```python
from build123d import *

# Parameters (mm, degrees)
SKETCH1_R           = 4.25
BOSS_EXTRUDE1_DEPTH = 20
SKETCH2_R           = 1
BOSS_EXTRUDE2_DEPTH = 0.5
SKETCH3_R           = 0.5
BOSS_EXTRUDE3_DEPTH = 5
FILLET2_R           = 0.5
FILLET3_R           = 0.1
FILLET4_R           = 0.5


with BuildPart() as part:
    # Sketch1 → Boss-Extrude1 (new body)
    with BuildSketch(Plane.XY):
        Circle(SKETCH1_R)
    extrude(amount=BOSS_EXTRUDE1_DEPTH)

    # Sketch2 → Boss-Extrude2 (add)
    with BuildSketch(Plane.XY.offset(20)):
        Circle(SKETCH2_R)
    extrude(amount=BOSS_EXTRUDE2_DEPTH)

    # Sketch3 → Boss-Extrude3 (add)
    with BuildSketch(Plane.XY.offset(20.5)):
        Circle(SKETCH3_R)
    extrude(amount=BOSS_EXTRUDE3_DEPTH)

    # Fillet2
    fillet2_edges = [part.edges().sort_by_distance(p)[0] for p in [
        (-4.25, 0, 20),
    ]]
    fillet(fillet2_edges, radius=FILLET2_R)

    # Fillet3
    fillet3_edges = [part.edges().sort_by_distance(p)[0] for p in [
        (-0.5, 0, 25.5),
    ]]
    fillet(fillet3_edges, radius=FILLET3_R)

    # Fillet4
    fillet4_edges = [part.edges().sort_by_distance(p)[0] for p in [
        (-4.25, 0, 0),
    ]]
    fillet(fillet4_edges, radius=FILLET4_R)


solid = part.part
```
Geometry check sheet. Reference: the model listing, model coordinates, mm. A direction names the side the tool comes from. Give positions to 0.01 mm unless a question says otherwise; leave off trailing zeros. Loops run counter-clockwise (first coordinate to the right, second up) from the corner with the lowest first, then second, coordinate; pieces in that order, holes last. Notation, with made-up numbers: M -31.5,60 L 24.5,60 A22 ccw 24.5,70 Z; hole C 2.25,70 d11. An arc over 180 degrees is marked long. Write item = value, one per line. Start each with the question number.
1. Thickness scan on probe 1 along Y at (x, z) = (-2, 12.75); probe 2 along Z at (x, y) = (0.5, 3.25); probe 3 along Y at (x, z) = (0, 24). Record the ranges inside material, lowest first.
2. Section check A-A, the plane x = 0. Enter the section's corners in (y, z).
3. Tool access check on faces 1 (the face through (2.285, 3.584, 9.867)), 2 (the face through (1, -1, 20)). Record the directions out of +Z, -Z, +X, -X, +Y, -Y that give a thin tool (end or side, any length) a straight path to the whole face; none if there is none.
4. Section check C-C, the plane z = 11. Enter the section's corners in (x, y), plus the area to 3 significant figures.
5. Go/stop test with flat-tipped pins: P1, Ø3, axis at x = -2.5, z = 9.5, coming from the +Y side; P2, Ø1.5, axis at y = -2, z = 18.5, coming from the -X side; P3, Ø2, axis at y = -3.5, z = 15, coming from the -X side. Record where each tip stops, or that it passes through.
Values follow:
q1.probe_1 = -3.75 to 3.75
q1.probe_2 = 0 to 20
q1.probe_3 = -0.5 to 0.5
q2.outline = M -4.25,0.5 A0.5 ccw -3.75,0 L 3.75,0 A0.5 ccw 4.25,0.5 L 4.25,19.5 A0.5 ccw 3.75,20 L 1,20 L 1,20.5 L 0.5,20.5 L 0.5,25.4 A0.1 ccw 0.4,25.5 L -0.4,25.5 A0.1 ccw -0.5,25.4 L -0.5,20.5 L -1,20.5 L -1,20 L -3.75,20 A0.5 ccw -4.25,19.5 Z
q3.face_1 = +Z, -Z
q3.face_2 = +Z
q4.outline = C 0,0 d8.5
q4.area = 56.7 mm^2
q5.P1 = 4.13
q5.P2 = -4.06
q5.P3 = -3.44
